For this review, take the finished solid that the model builds, in its own axes (mm). Coordinates: 2 decimals unless noted, no trailing zeros. Loops run counter-clockwise (first coordinate to the right, second up) from the corner with the lowest first, then second, coordinate; pieces in that order, holes last. Notation, with made-up numbers: (-12, 43) - (31, 43) arc R9 ccw to (31, 53) - close; hole circle Ø2 at (57, -3.5). An arc over 180 degrees is marked (long way). Use one line per item in the form item = value. Start each with the question number.
1. To check wall thickness, follow probe 1 along Z at (x, y) = (50.5, 82.5); probe 2 along Z at (x, y) = (26, 241.5). State the ranges of each line that lie inside material, in increasing order.
2. For pin 1 Ø10 at (x, y) = (20.5, 215.5) entering from +Z; pin 2 Ø6 at (x, y) = (20, 296.5) entering from -Z; pin 3 Ø12 at (x, y) = (71, 164.5) entering from +Z, all flat-tipped, find the tip position at first contact; note any pin that passes through.
3. Add section A-A on x = 75. Give the boundary of the cut face in (y, z).
```python
from build123d import *

# Parameters (mm, degrees)
F0_W     = 100
F0_H     = 135
F0_W_2   = 60
F0_H_2   = 120
F1_DEPTH = 100
F2_R     = 2.5


with BuildPart() as f1:
    # F0 (on Right) → F1 (new body)
    with BuildSketch(Plane.YZ):
        Rectangle(F0_W, F0_H)
        Polygon((430, 60), (50, 67.5), (50, -67.5), (430, -60), (370, -60), (370, 60), align=None)
        with Locations((400, 0)):
            Rectangle(F0_W_2, F0_H_2)
    extrude(amount=F1_DEPTH)

    # F2
    f2_edges = [f1.edges().sort_by_distance(p)[0] for p in [
        (100, 240, 63.75),
        (100, 430, 0),
        (100, 240, -63.75),
        (100, 0, 67.5),
        (100, -50, 0),
        (100, 0, -67.5),
        (50, -50, -67.5),
        (0, -50, 0),
        (0, 0, 67.5),
        (0, 240, -63.75),
        (0, 0, -67.5),
        (50, 430, -60),
        (0, 430, 0),
        (50, 430, 60),
        (0, 240, 63.75),
        (50, -50, 67.5),
    ]]
    fillet(f2_edges, radius=F2_R)


solid = f1.part
```
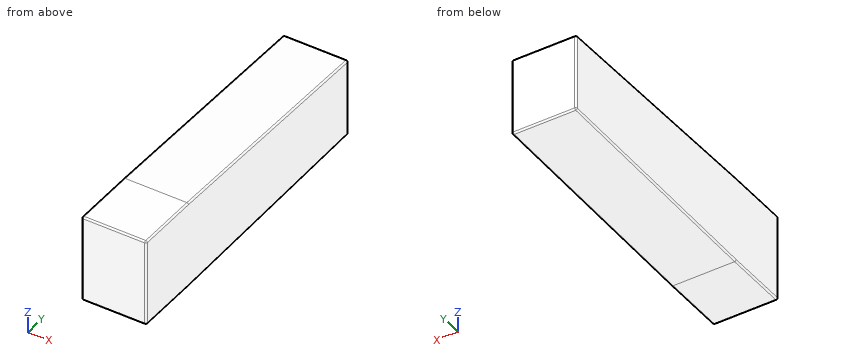
Conclusion:
q1.probe_1 = -66.86 to 66.86
q1.probe_2 = -63.72 to 63.72
q2.pin_1 = 64.33
q2.pin_2 = -62.69
q2.pin_3 = 65.36
q3.outline = (-50, -65) arc R2.5 ccw to (-47.5, -67.5) - (50, -67.5) - (427.55, -60.05) arc R2.5 ccw to (430, -57.55) - (430, 57.55) arc R2.5 ccw to (427.55, 60.05) - (50, 67.5) - (-47.5, 67.5) arc R2.5 ccw to (-50, 65) - close
